Here's the drawing with two shaded views (mm, measured from the low corner). I have some questions. A direction names the side the tool comes from. Round coordinates to 2 decimals unless told otherwise and drop trailing zeros. Order: outer loops, then holes, each group sorted by start corner. A loop starts at its lowest first (then second) coordinate and runs counter-clockwise, first axis right, second up. Notation, with made-up numbers: (45, 28.5) -> (102, 28.5) arc R16 cw to (102, 53.5) -> close; hole circle Ø1 at (-21.5, -31). An arc over 180 degrees is marked (long way). Put each result on its own line as item: value. Start each with the question number.
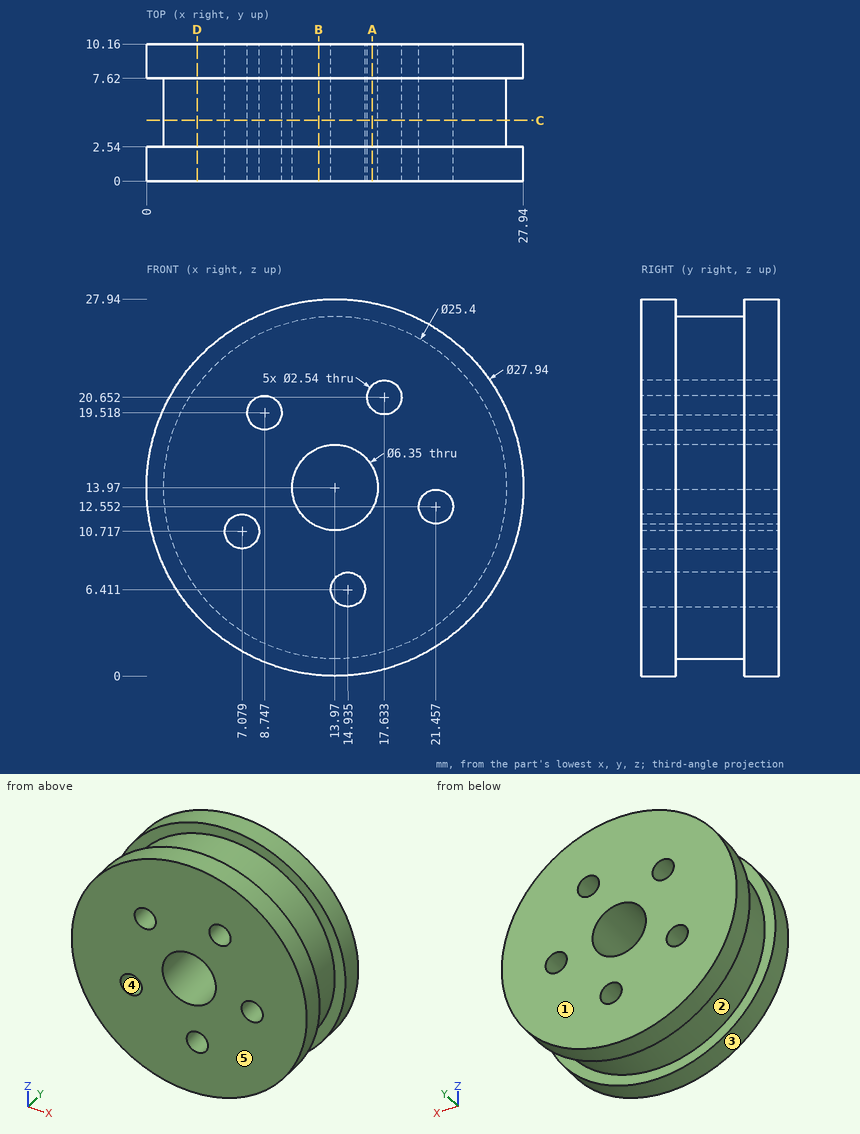
1. Which directions (+Z, -Z, +X, -X, +Y, -Y) give clear straight access to the entire face, cutting with the end or side of a thin tool? Please do the marked faces 1 and 2.
2. If we section it at B-B, the plane x = 12.75: Please give me the cut outline in (y, z).
3. Thinking about a two-plate mould opening in X: for the marked faces 3, 4 and 5, which applies, +X half, -X half, draft (parallel to the pull), parting line (faces both ways), or undercut?
4. If we section it at C-C, the plane y = 4.5: Count the separate pieces of the cut face and the enclosed holes in it, then the cut area to 3 significant figures.
5. For pin 1 Ø1 at (x, y) = (7.5, 9) entering from -Z; pin 2 Ø1.5 at (y, z) = (2, 8.5) entering from -X; pin 3 Ø4 at (x, y) = (8.5, 6) entering from -Z, each with a flat end and sliding along its axis, tell me the tip position at first contact or that it passes through.
6. If we section it at D-D, the plane x = 3.75: Please give me the cut outline in (y, z) (1 decimal).
7. If we section it at A-A, the plane x = 16.75: Please give me the cut outline in (y, z) (1 decimal), then the cut area to 3 significant figures.
8. I need wall thicknesses on L1, parallel to Y at x = 18.5, z = 2; L2, parallel to X at y = 3.75, z = 11.25 (1 decimal); L3, parallel to X at y = 4.25, z = 13.97 (1 decimal). Which ranges of each line are inside material? Lowest first, please.
Results below:
1. face 1: +Z, -Z, +X, -X, +Y
1. face 2: none
2. outline: (0, 0.05) -> (2.54, 0.05) -> (2.54, 1.33) -> (7.62, 1.33) -> (7.62, 0.05) -> (10.16, 0.05) -> (10.16, 11.04) -> (0, 11.04) -> close; (0, 16.9) -> (10.16, 16.9) -> (10.16, 27.89) -> (7.62, 27.89) -> (7.62, 26.61) -> (2.54, 26.61) -> (2.54, 27.89) -> (0, 27.89) -> close
3. face 3: parting line
3. face 4: undercut
3. face 5: draft
4. separate pieces: 1
4. enclosed holes: 6
4. area: 450 mm2
5. pin 1: z = 1.34
5. pin 2: x = 0.82
5. pin 3: z = 0.68
6. outline: (0, 4.4) -> (2.5, 4.4) -> (2.5, 6.4) -> (7.6, 6.4) -> (7.6, 4.4) -> (10.2, 4.4) -> (10.2, 23.5) -> (7.6, 23.5) -> (7.6, 21.5) -> (2.5, 21.5) -> (2.5, 23.5) -> (0, 23.5) -> close
7. outline: (0, 0.3) -> (2.5, 0.3) -> (2.5, 1.6) -> (7.6, 1.6) -> (7.6, 0.3) -> (10.2, 0.3) -> (10.2, 12.4) -> (0, 12.4) -> close; (0, 15.5) -> (10.2, 15.5) -> (10.2, 19.7) -> (0, 19.7) -> close; (0, 21.6) -> (10.2, 21.6) -> (10.2, 27.7) -> (7.6, 27.7) -> (7.6, 26.4) -> (2.5, 26.4) -> (2.5, 27.7) -> (0, 27.7) -> close
7. area: 215 mm2
8. L1: 0 to 2.54, 7.62 to 10.16
8. L2: 1.6 to 5.9, 8.2 to 12.3, 15.6 to 26.4
8. L3: 1.3 to 10.8, 17.1 to 26.7
